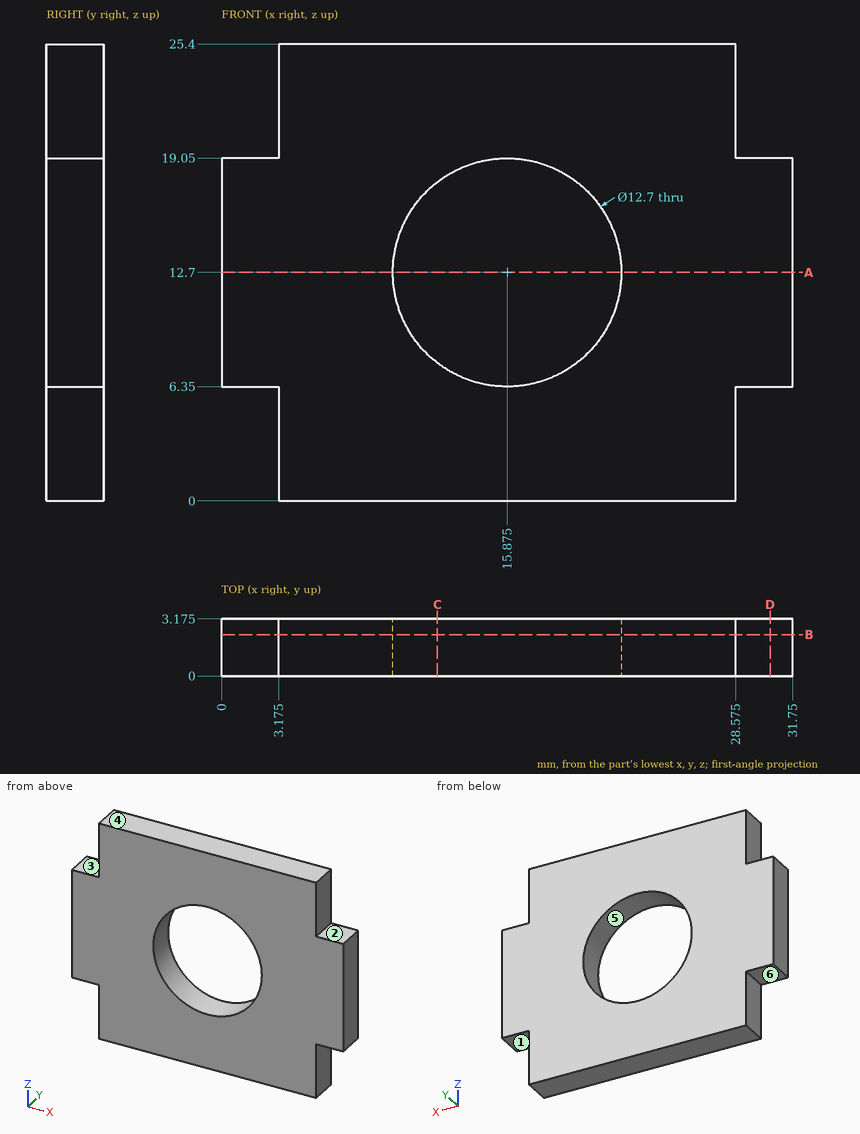
Study the drawing (mm; zero at the part's minimum x, y, z) and answer. A direction names the side the tool comes from. Give positions to 0.01 mm unless a question says otherwise; leave off trailing zeros. Write each loop counter-clockwise with the first axis right and the second up, starting at its lowest first coordinate (ties: lowest second). Pieces come first, ordered by that corner, then holes. Notation, with made-up numbers: (84.5, 25) -> (129.5, 25) arc R12 cw to (129.5, 48) -> close; hole circle Ø11 at (16.5, 87). An arc over 180 degrees is marked (long way). Write item = value, one per line. Start each with the question number.
1) Which of the six approach directions +Z, -Z, +X, -X, +Y, -Y give full straight-line access (tool end or side, diameter ignored) to the marked faces 1, 2 and 3?
2) The part is cut by section A-A, the plane z = 12.7. Determine the outline of the cut face in (x, y) (3 decimals), and give its area (3 significant figures).
3) Each of these flat-tipped pins is pushed along its axis until it touches: pin 1 (1.6 mm diameter, centred on y = 1, z = 22.5, fed in from -X) (3 decimals); pin 2 (1 mm diameter, centred on x = 2.5, y = 1, fed in from +Z). Where does it stop, or does it pass through?
4) Straight lines are drawn through the part: line 1 along X through (y, z) = (2.55, 12.5); line 2 along Z through (x, y) = (20, 1.7); line 3 along X through (y, z) = (0.8, 23.75) (3 decimals). For each, find the intervals that lie inside material, in ascending order.
5) The part is cut by section B-B, the plane y = 2.3. Determine the outline of the cut face in (x, z) (3 decimals).
6) The part is cut by section C-C, the plane x = 12. Determine the outline of the cut face in (y, z) (3 decimals).
7) The part is cut by section D-D, the plane x = 30.5. Determine the outline of the cut face in (y, z) (3 decimals), and give its area (3 significant figures).
8) Determine the mould class of the marked faces 4, 5 and 6 for opening direction Z: +Z half, -Z half, draft (parallel to the pull), parting line (faces both ways), or undercut.
Solutions:
q1.face_1 = -Z, +X, +Y, -Y
q1.face_2 = +Z, +X, +Y, -Y
q1.face_3 = +Z, -X, +Y, -Y
q2.outline = (0, 0) -> (9.525, 0) -> (9.525, 3.175) -> (0, 3.175) -> close; (22.225, 0) -> (31.75, 0) -> (31.75, 3.175) -> (22.225, 3.175) -> close
q2.area = 60.5 mm²
q3.pin_1 = 3.175
q3.pin_2 = 19.05
q4.line_1 = 0 to 9.53, 22.22 to 31.75
q4.line_2 = 0 to 7.87, 17.53 to 25.4
q4.line_3 = 3.175 to 28.575
q5.outline = (0, 6.35) -> (3.175, 6.35) -> (3.175, 0) -> (28.575, 0) -> (28.575, 6.35) -> (31.75, 6.35) -> (31.75, 19.05) -> (28.575, 19.05) -> (28.575, 25.4) -> (3.175, 25.4) -> (3.175, 19.05) -> (0, 19.05) -> close; hole circle Ø12.7 at (15.875, 12.7)
q6.outline = (0, 0) -> (3.175, 0) -> (3.175, 7.669) -> (0, 7.669) -> close; (0, 17.731) -> (3.175, 17.731) -> (3.175, 25.4) -> (0, 25.4) -> close
q7.outline = (0, 6.35) -> (3.175, 6.35) -> (3.175, 19.05) -> (0, 19.05) -> close
q7.area = 40.3 mm²
q8.face_4 = +Z half
q8.face_5 = undercut
q8.face_6 = -Z half
